from build123d import *

# Parameters (mm, degrees)
F1_DEPTH = 2.5


# Not quite as in the source:
# - a feature names something its author has since deleted; it is built from what else it names


with BuildPart() as f1:
    # F0 (on Front) → F1 (new body)
    with BuildSketch(Plane.XZ):
        with BuildLine():
            Line((-16.7953648853, -9.0339062735), (-6.5833406376, -9.0339062735))
            Line((-6.5833406376, -9.0339062735), (-3, -9.0339062735))
            Line((-3, -9.0339062735), (-3, -10.7153228952))
            Line((-3, -10.7153228952), (-1.9461073071, -10.7153228952))
            ThreePointArc((-1.9461073071, -10.7153228952), (-0.5700016333, -10.1453212619), (0, -8.7692155881))
            Line((0, -8.7692155881), (0, -8.5))
            Line((0, -8.5), (0, -7.5339062735))
            Line((0, -7.5339062735), (-10, -7.5339062735))
            Line((-10, -7.5339062735), (-10, -2.6866213954))
            Line((-10, -2.6866213954), (0.2046351147, -2.6866213954))
            Line((0.2046351147, -2.6866213954), (0.2046351147, -1.7576624442))
            Line((0.2046351147, -1.7576624442), (0.2046351147, -1.4884468561))
            ThreePointArc((0.2046351147, -1.4884468561), (-0.3653665186, -0.1123411824), (-1.7414721924, 0.457660451))
            Line((-1.7414721924, 0.457660451), (-2.7953648853, 0.457660451))
            Line((-2.7953648853, 0.457660451), (-2.7953648853, -1.1866213954))
            Line((-2.7953648853, -1.1866213954), (-6.7360828114, -1.1866213954))
            Line((-6.7360828114, -1.1866213954), (-16.7953648853, -1.1866213954))
            Line((-16.7953648853, -1.1866213954), (-16.7953648853, -9.0339062735))
        make_face()
    extrude(amount=F1_DEPTH)


solid = f1.part
CAD build for the part. Positions are in the model's coordinates, mm. A direction names the side the tool comes from. Round coordinates to 2 decimals unless told otherwise and drop trailing zeros. Write each loop counter-clockwise with the first axis right and the second up, starting at its lowest first coordinate (ties: lowest second). Pieces come first, ordered by that corner, then holes. Notation, with made-up numbers: M -7.5,-20 L 37.5,-20 A36 cw 37.5,18 Z; hole C -8,38 d8. An arc over 180 degrees is marked long. Put each result on its own line as item: value. Start each with the question number.
1) 3-axis set-ups, long thin cutter, end or side, ignore diameter. For faces 1 (the flat face through (-2.5, -1.2, -10.715)), 2 (the flat face through (-10, -1, -1.187)), 3 (the flat face through (0, -1, -8)), 4 (the flat face through (-10, -1, -5)), 5 (the flat face through (-10, -1, -9.034)): which of +Z, -Z, +X, -X, +Y, -Y reach the whole face in a straight line?
2) Pin check, flat tips, straight feed: pin 1 Ø1.4 at (y, z) = (-1.5, -8) entering from +X; pin 2 Ø0.8 at (x, y) = (-13, -1) entering from -Z; pin 3 Ø1.5 at (y, z) = (-0.5, -6) entering from +X. Stop position of each tip, or through.
3) Saw through at B-B, the plane y = -1.5. Write the cut outline in (x, z).
4) Drill centre lines: probe 1 along Z at (x, y) = (-9.5, -1.75); probe 2 along X at (y, z) = (-1.75, -8.25); probe 3 along X at (y, z) = (-2.05, -6). Where is each one in solid material? Low to high. Write a range as [from, to].
5) Saw through at A-A, the plane x = -6. Write the cut outline in (y, z), and give its area (3 significant figures).
6) Saw through at D-D, the plane x = -1.5. Write the cut outline in (y, z), and give its area (3 significant figures).
7) Saw through at C-C, the plane z = -3. Write the cut outline in (x, y), and give its area (3 significant figures).
8) Pull direction Z, two halves, no side cores. Call faces 6 (the flat face through (-5, -1, -2.687)), 7 (the cylindrical face through (-0.585, -1.232, -10.16)), 8 (the flat face through (-2, -1, 0.458)): pulls with the +Z half, pulls with the -Z half, needs draft (parallel to the pull), parting line crosses it, or undercut.
Resolved:
1. face 1: -Z, +X, -X, +Y, -Y
1. face 2: +Z, -X, +Y, -Y
1. face 3: -Z, +X, +Y, -Y
1. face 4: +X, +Y, -Y
1. face 5: -Z, -X, +Y, -Y
2. pin 1: x = 0
2. pin 2: z = -9.03
2. pin 3: x = -10
3. outline: M -16.8,-9.03 L -3,-9.03 L -3,-10.72 L -1.95,-10.72 A1.95 ccw 0,-8.77 L 0,-7.53 L -10,-7.53 L -10,-2.69 L 0.2,-2.69 L 0.2,-1.49 A1.95 ccw -1.74,0.46 L -2.8,0.46 L -2.8,-1.19 L -16.8,-1.19 Z
4. probe 1: [-9.03, -7.53], [-2.69, -1.19]
4. probe 2: [-16.8, 0]
4. probe 3: [-16.8, -10]
5. outline: M -2.5,-9.03 L 0,-9.03 L 0,-7.53 L -2.5,-7.53 Z; M -2.5,-2.69 L 0,-2.69 L 0,-1.19 L -2.5,-1.19 Z
5. area: 7.50 mm²
6. outline: M -2.5,-10.66 L 0,-10.66 L 0,-7.53 L -2.5,-7.53 Z; M -2.5,-2.69 L 0,-2.69 L 0,0.44 L -2.5,0.44 Z
6. area: 15.6 mm²
7. outline: M -16.8,-2.5 L -10,-2.5 L -10,0 L -16.8,0 Z
7. area: 17.0 mm²
8. face 6: undercut
8. face 7: pulls with the -Z half
8. face 8: pulls with the +Z half
